```python
from build123d import *

# Parameters (mm, degrees)
BOSS_EXTRUDE1_DEPTH                    = 80
SKETCH2_W                              = 127.893941609
SKETCH2_H                              = 47.2063817
CUT_EXTRUDE1_DEPTH                     = 50
FILLET1_R                              = 6
CBORE_FOR_M6_HEX_HEAD_BOLT1_AT_2_COUNT = 2
CBORE_FOR_M6_HEX_HEAD_BOLT1_AT_2_PITCH = 50


with BuildPart() as part:
    # Sketch1 → Boss-Extrude1 (new body)
    with BuildSketch(Plane(origin=(0, 0, 0), x_dir=(1, 0, 0), z_dir=(0, 1, 0))):
        Polygon((-20, -57), (-20, -35), (20, -35), (20, -57), (23, -60), (52, -60), (55, -57), (55, 0), (-55, 0), (-55, -57), (-52, -60), (-23, -60), align=None)
    extrude(amount=BOSS_EXTRUDE1_DEPTH)

    # Sketch2 → Cut-Extrude1 (cut)
    with BuildSketch(Plane(origin=(0, 80, 0), x_dir=(1, 0, 0), z_dir=(0, 1, 0))):
        with Locations((-0.415915258, -48.60319085)):
            Rectangle(SKETCH2_W, SKETCH2_H)
    extrude(amount=-CUT_EXTRUDE1_DEPTH, mode=Mode.SUBTRACT)

    # Fillet1
    fillet1_edges = [part.edges().sort_by_distance(p)[0] for p in [
        (55, 80, 12.5),
        (-55, 80, 12.5),
    ]]
    fillet(fillet1_edges, radius=FILLET1_R)

    # Sketch3 → CBORE for M6 Hex Head Bolt1 (revolve, cut)
    with BuildSketch(Plane(origin=(-25, 55, 25), x_dir=(0, -1, 0), z_dir=(1, 0, 0))):
        Polygon((0, 0), (0, 25), (3.2, 25), (3.2, 9.38), (7.275, 9.38), (7.275, 0.025), (7.3, 0), align=None)
    cbore_for_m6_hex_head_bolt1 = revolve(axis=Axis((-25, 55, 31.35), (0, 0, -1)), mode=Mode.SUBTRACT)

    # CBORE for M6 Hex Head Bolt1 at 2: CBORE for M6 Hex Head Bolt1 ×2
    with Locations(*[(i * CBORE_FOR_M6_HEX_HEAD_BOLT1_AT_2_PITCH, 0, 0) for i in range(1, CBORE_FOR_M6_HEX_HEAD_BOLT1_AT_2_COUNT)]):
        add(cbore_for_m6_hex_head_bolt1, mode=Mode.SUBTRACT)


solid = part.part
```
Geometry check sheet. Reference: the model listing, model coordinates, mm. A direction names the side the tool comes from. Round coordinates to 2 decimals unless told otherwise and drop trailing zeros. Order: outer loops, then holes, each group sorted by start corner. A loop starts at its lowest first (then second) coordinate and runs counter-clockwise, first axis right, second up. Notation, with made-up numbers: (75, -13.5) -> (118, -13.5) arc R31 ccw to (118, 18.5) -> close; hole circle Ø1 at (27.5, -37). An arc over 180 degrees is marked (long way). Return JSON: item names as keys, results as strings. Group by question number.
Q1. Gauge pin test, flat ends, axial feed: pin 1 (9 mm diameter, centred on x = -3.5, y = 8.5, fed in from +Z); pin 2 (11.5 mm diameter, centred on x = 25, y = 55, fed in from +Z); pin 3 (25 mm diameter, centred on x = 13.5, y = 52.5, fed in from +Z). Record the tip position at first contact, or that the pin passes through.
Q2. Section check A-A, the plane y = 55. Record the boundary of the cut face in (x, z) (3 decimals), plus the area to 3 significant figures.
Q3. Section check D-D, the plane z = 44.5. Record the boundary of the cut face in (x, y).
Q4. Section check B-B, the plane x = 25. Record the boundary of the cut face in (y, z) (3 decimals), plus the area to 3 significant figures.
Q5. Release check for a two-part mould opening along Y. For faces 4 (the flat face through (-54, 15, 58)), 5 (the flat face through (-1, 0, 30)), 6 (the cylindrical face through (26.947, 57.539, 7.919)), 7 (the cylindrical face through (-25.1, 58.2, 7.9)) record: released by +Y, released by -Y, zero draft, split by the parting line, or undercut.
Q6. Tool access check on faces 1 (the flat face through (-22, 15, 59)), 2 (the cylindrical face through (22.815, 48.061, 20.363)), 3 (the flat face through (-1, 55, 25)). Record the directions out of +Z, -Z, +X, -X, +Y, -Y that give a thin tool (end or side, any length) a straight path to the whole face; none if there is none.
Q7. Material ranges on probe 1 along X at (y, z) = (55, 23) (3 decimals); probe 2 along X at (y, z) = (55, 10.75); probe 3 along Y at (x, z) = (25, 18.75) (3 decimals), recorded low to high. Write a range as from..to.
Q8. Section check C-C, the plane z = 23. Record the boundary of the cut face in (x, y) (3 decimals).
Numbers:
{
 "1": {"pin 1": "z = 35", "pin 2": "z = 15.62", "pin 3": "z = 25"},
 "2": {"outline": "(-55, 0) -> (-28.2, 0) -> (-28.2, 15.62) -> (-32.275, 15.62) -> (-32.275, 24.975) -> (-32.3, 25) -> (-55, 25) -> close; (-21.8, 0) -> (21.8, 0) -> (21.8, 15.62) -> (17.725, 15.62) -> (17.725, 24.975) -> (17.7, 25) -> (-17.7, 25) -> (-17.725, 24.975) -> (-17.725, 15.62) -> (-21.8, 15.62) -> close; (28.2, 0) -> (55, 0) -> (55, 25) -> (32.3, 25) -> (32.275, 24.975) -> (32.275, 15.62) -> (28.2, 15.62) -> close", "area": "2,280 mm^2"},
 "3": {"outline": "(-55, 0) -> (-20, 0) -> (-20, 30) -> (-55, 30) -> close; (20, 0) -> (55, 0) -> (55, 30) -> (20, 30) -> close"},
 "4": {"outline": "(0, 0) -> (51.8, 0) -> (51.8, 15.62) -> (47.725, 15.62) -> (47.725, 24.975) -> (47.7, 25) -> (30, 25) -> (30, 60) -> (0, 60) -> close; (58.2, 0) -> (80, 0) -> (80, 25) -> (62.3, 25) -> (62.275, 24.975) -> (62.275, 15.62) -> (58.2, 15.62) -> close", "area": "2,810 mm^2"},
 "5": {"face 4": "zero draft", "face 5": "released by -Y", "face 6": "undercut", "face 7": "undercut"},
 "6": {"face 1": "+Z, +Y, -Y", "face 2": "+Z", "face 3": "+Z, +X, -X, +Y"},
 "7": {"probe 1": "-55..-32.275, -17.725..17.725, 32.275..55", "probe 2": "-55..-28.2, -21.8..21.8, 28.2..55", "probe 3": "0..47.725, 62.275..80"},
 "8": {"outline": "(-55, 0) -> (55, 0) -> (55, 74) arc R6 ccw to (49, 80) -> (-49, 80) arc R6 ccw to (-55, 74) -> close; hole circle Ø14.55 at (-25, 55); hole circle Ø14.55 at (25, 55)"}
}
